Part model, mm, in its own coordinate system. Round coordinates to 2 decimals unless told otherwise and drop trailing zeros. Return JSON: item names as keys, results as strings. Group by question number.
Autodesk Inventor part; units mm, degrees
ref_plane "Work Plane1" through (0, 4.7625, 0) normal (0, 1, 0) x (1, 0, 0)
ref_plane "YZ Plane" through (0, 0, 0) normal (1, 0, 0) x (0, 1, 0)
ref_plane "XZ Plane" through (0, 0, 0) normal (0, 1, 0) x (-1, 0, 0)
sketch "Sketch1" plane through (0, 0, 0) normal (0, 1, 0) x (-1, 0, 0)
  circle A0 centre (0, 0) radius 22.225 construction
  circle A1 centre (0, 0) radius 17.65
  circle A2 centre (0, 0) radius 24.3125
  dimension "d0" = 44.45
  dimension "d1" = 35.3
  dimension "d2" = 48.625
extrude "Extrusion1" add sketch "Sketch1" along normal blind 9.525
sketch "Sketch2" plane through (0, 0, 0) normal (0, -1, 0) x (1, 0, 0)
  circle A0 centre (0, 0) radius 17.6
  circle A1 centre (0, 0) radius 20.6375
  dimension "d5" = 41.275
  dimension "d6" = 35.2
extrude "Extrusion2" add sketch "Sketch2" along normal blind 1.5875
sketch "Sketch3" plane through (0, 9.525, 0) normal (0, 1, 0) x (1, 0, 0)
  circle A0 centre (0, 0) radius 17.65
  circle A1 centre (0, 0) radius 19.8438
  dimension "d9" = 35.3
  dimension "d10" = 39.6875
extrude "Extrusion3" add sketch "Sketch3" along normal blind 1.5875
sketch "Sketch4" plane through (0, 0, 0) normal (1, 0, 0) x (0, 1, 0)
  line L0 (11.1125, -17.65) -> (17.8875, -17.65)
  line L1 (17.8875, -17.65) -> (17.8875, -20.6375)
  line L2 (17.8875, -20.6375) -> (11.1125, -20.6375) construction
  line L3 (11.1125, -20.6375) -> (11.1125, -17.65)
  line L4 (11.1125, -19.8438) -> (11.1125, 19.8438)
  line L5 (12.7, -17.65) -> (12.7, -20.6375) construction
  line L6 (11.1125, -19.8438) -> (12.7, -19.8438)
  line L7 (12.7, -19.8438) -> (17.8875, -19.8438)
  line L8 (0, 0) -> (25.7056, 0) construction
  line L9 (-11.1125, 0) -> (-11.1125, -19.8438) construction
  line L10 (0, 20.6375) -> (0, -20.6375)
  dimension "d13" = 17.65
  dimension "d14" = 20.6375
  dimension "d16" = 1.5875
  dimension "d18" = 19.8438
  dimension "d84" = 11.1125
  dimension "d85" = 29
revolve "Revolution1" add sketch "Sketch4" angle 360 about axis through (0, 0, 0) along (0, 1, 0)
ref_plane "Work Plane1" through (0, 4.7625, 0) normal (0, 1, 0) x (1, 0, 0)
sketch "Sketch11" plane through (0, 17.8875, 0) normal (0, 1, 0) x (1, 0, 0)
  circle A0 centre (0, 0) radius 11.75 construction
  line L0 (0, 0) -> (-11.75, 0) construction
  circle A1 centre (-11.75, 0) radius 3.875
  line L1 (-11.75, -3.875) -> (-18.1, -3.875)
  line L2 (-18.1, -3.875) -> (-18.1, 3.875)
  line L3 (-18.1, 3.875) -> (-11.75, 3.875)
  line L4 (-11.75, 3.875) -> (-11.75, -3.875) construction
  circle A2 centre (0, -11.75) radius 3.875
  line L5 (3.875, -11.75) -> (3.875, -18.1)
  line L6 (3.875, -18.1) -> (-3.875, -18.1)
  line L7 (-3.875, -18.1) -> (-3.875, -11.75)
  line L8 (-3.875, -11.75) -> (3.875, -11.75) construction
  circle A3 centre (11.75, 0) radius 3.875
  line L9 (11.75, 3.875) -> (18.1, 3.875)
  line L10 (18.1, 3.875) -> (18.1, -3.875)
  line L11 (18.1, -3.875) -> (11.75, -3.875)
  line L12 (11.75, -3.875) -> (11.75, 3.875) construction
  circle A4 centre (0, 11.75) radius 3.875
  line L13 (-3.875, 11.75) -> (-3.875, 18.1)
  line L14 (-3.875, 18.1) -> (3.875, 18.1)
  line L15 (3.875, 18.1) -> (3.875, 11.75)
  line L16 (3.875, 11.75) -> (-3.875, 11.75) construction
  circle A5 centre (0, -11.75) radius 1.7526
  circle A6 centre (11.75, 0) radius 1.7526
  circle A7 centre (0, 11.75) radius 1.7526
  circle A8 centre (-11.75, 0) radius 1.7526
  point P0 (3.875, 11.75)
  point P1 (11.75, -3.875)
  point P2 (-3.875, -11.75)
  point P3 (-11.75, 3.875)
  dimension "d121" = 23.5
  dimension "d122" = 7.75
  dimension "d123" = 6.35
  dimension "d126" = 360
  dimension "d134" = 3.5052
  dimension "d137" = 360
extrude "Extrusion10" add sketch "Sketch11" against normal blind 3
fillet "Fillet5" radius 0.5 8 edges at (-17.2194, 16.3875, -3.875) (-17.2194, 16.3875, 3.875) (-3.875, 16.3875, 17.2194) (3.875, 16.3875, 17.2194) (17.2194, 16.3875, -3.875) (17.2194, 16.3875, 3.875) (-3.875, 16.3875, -17.2194) (3.875, 16.3875, -17.2194)
chamfer "Chamfer5" distance 1.5875 angle 45 1 edges at (-17.6, -1.5875, 0)
chamfer "Chamfer6" distance 1.5875 angle 45 2 edges at (24.3125, 9.525, 0) (24.3125, 0, 0)
chamfer "Chamfer8" distance 2.3813 angle 45 1 edges at (-19.8438, 9.525, 0)
properties part number "Motor Hub" material "Nylon 6/6"
(1) Probe L1, parallel to Z at x = 0, y = 15.75 (3 decimals); L2, parallel to X at y = 13.5, z = 0. List the from-to ranges inside material, lowest first. Write a range as [from, to].
(2) Pin check, flat tips, straight feed: P1, Ø7, axis at x = 1, z = 13, coming from the -Y side; P2, Ø2, axis at y = 4, z = 15.5, coming from the +X side; P3, Ø22.5, axis at x = 2.5, z = -1, coming from the +Y side; P4, Ø8, axis at y = 15, z = 1.5, coming from the -X side. Stop position of each tip, or through.
(3) Saw through at A-A, the plane z = 0. State how many separate pieces and enclosed holes the cut face has, and give its area (3 significant figures).
(4) Mould opens along Z. For faces 1 (the flat face through (14, -1.588, -14)), 2 (the cylindrical face through (-0.228, 16.408, -13.488)), 3 (the cylindrical face through (-4.474, -0.783, 20.147)) say: pulls with the +Z half, pulls with the -Z half, needs draft (parallel to the pull), parting line crosses it, or undercut.
Results are:
{
 "1": {"L1": "z = [-19.844, -13.503], [-9.997, -7.875], [7.875, 9.997], [13.503, 19.844]", "L2": "x = [-19.84, -17.65], [17.65, 19.84]"},
 "2": {"P1": "stops at y = 14.89", "P2": "stops at x = 19.52", "P3": "stops at y = 17.89", "P4": "stops at x = -20.7"},
 "3": {"separate pieces": "4", "enclosed holes": "0", "area": "209 mm^2"},
 "4": {"face 1": "needs draft", "face 2": "undercut", "face 3": "parting line crosses it"}
}
